```python
from build123d import *

# Parameters (mm, degrees)
SKETCH1_W                = 150
SKETCH1_H                = 12
BOSS_EXTRUDE1_DEPTH      = 20
SKETCH2_R                = 20
SKETCH2_R_2              = 10
BOSS_EXTRUDE2_DEPTH      = 30
FILLET1_R                = 10
SKETCH3_W                = 10
SKETCH3_H                = 80
BOSS_EXTRUDE3_DEPTH      = 15
BOSS_EXTRUDE4_DEPTH      = 40
BOSS_EXTRUDE4_DEPTH_BACK = 20
SKETCH4_R                = 15
SKETCH4_R_2              = 7.5
RIB1_START               = -5
RIB1_DEPTH               = 10


# Read off the part's stored shape, not the designer's step: Rib1
with BuildPart() as part:
    # Sketch1 → Boss-Extrude1 (new, symmetric)
    with BuildSketch(Plane.YZ):
        with Locations((75, 6)):
            Rectangle(SKETCH1_W, SKETCH1_H)
    extrude(amount=BOSS_EXTRUDE1_DEPTH, both=True)

    # Sketch2 → Boss-Extrude2 (add, symmetric)
    with BuildSketch(Plane.YZ):
        with Locations(Location((100, 30, 0), (0, 0, 270))):
            Circle(SKETCH2_R)
        with Locations(Location((100, 30, 0), (0, 0, 270))):
            Circle(SKETCH2_R_2, mode=Mode.SUBTRACT)
    extrude(amount=BOSS_EXTRUDE2_DEPTH, both=True)

    # Fillet1
    fillet1_edges = [part.edges().sort_by_distance(p)[0] for p in [
        (0, 108.717797887, 12),
    ]]
    fillet(fillet1_edges, radius=FILLET1_R)

    # Sketch3 → Boss-Extrude3 (add, symmetric)
    with BuildSketch(Plane.YZ):
        with Locations((35, 52)):
            Rectangle(SKETCH3_W, SKETCH3_H)
    extrude(amount=BOSS_EXTRUDE3_DEPTH, both=True)

    # Sketch4 → Boss-Extrude4 (add, two sides: drawn at the far end of the back side and taken through both)
    with BuildSketch(Plane(origin=(0, 40, 0), x_dir=(-1, 0, 0), z_dir=(0, 1, 0)).offset(-BOSS_EXTRUDE4_DEPTH_BACK)):
        with Locations(Location((0, 92, 0), (0, 0, 90))):
            Circle(SKETCH4_R)
        with Locations(Location((0, 92, 0), (0, 0, 90))):
            Circle(SKETCH4_R_2, mode=Mode.SUBTRACT)
    extrude(amount=BOSS_EXTRUDE4_DEPTH + BOSS_EXTRUDE4_DEPTH_BACK)

    # Rib1 outline → Rib1 (add)
    with BuildSketch(Plane.YZ.offset(RIB1_START)):
        with BuildLine():
            ThreePointArc((85, 50), (81.464466094, 51.464466094), (80, 55))
            Line((80, 55), (80, 79))
            Line((80, 79), (40, 79))
            Line((40, 79), (40, 12))
            Line((40, 12), (91.282202113, 12))
            ThreePointArc((91.282202113, 12), (80.50641131, 34.472135955), (100, 50))
            Line((100, 50), (85, 50))
        make_face()
    extrude(amount=RIB1_DEPTH)


solid = part.part
```
Geometry: final body of the model. Coordinates: model frame, mm. A direction names the side the tool comes from. Give positions to 0.01 mm unless a question says otherwise; leave off trailing zeros. Order: outer loops, then holes, each group sorted by start corner. A loop starts at its lowest first (then second) coordinate and runs counter-clockwise, first axis right, second up. Notation, with made-up numbers: (74, -34.5) -> (88, -34.5) arc R26 cw to (88, -18.5) -> close; hole circle Ø4 at (89.5, 62). An arc over 180 degrees is marked (long way). Write each question's results on one line, items separated by ' | '. Start each with the question number.
1) Section B-B (x = 0). Return loops of the section in (y, z).
2) Section D-D (z = 67). Return loops of the section in (x, y), then the cut area to 3 significant figures.
3) Line query: line 1 (Y direction, x = -8, z = 30); line 2 (Z direction, x = 0, y = 67); line 3 (X direction, y = 62.5, z = 92). Output: solid intervals per line, ascending. Write a range as from..to.
4) Section C-C (y = 76). Return loops of the section in (x, z), then the cut area to 3 significant figures.
5) Section A-A (y = 24). Return loops of the section in (x, z), then the cut area to 3 significant figures.
6) Set-up query: faces 4 (the cylindrical face through (-5.745, 49.58, 105.856)), 5 (the flat face through (10, 40, 51)), 6 (the flat face through (-15, 35, 53)), 7 (the flat face through (0, 35, 92)), 8 (the flat face through (0, 93, 50)). Return all of +Z, -Z, +X, -X, +Y, -Y with unobstructed straight access to the full face (end or side cutting, diameter ignored); none if empty.
7) Draft query along Y for faces 1 (the flat face through (15, 35, 53)), 2 (the cylindrical face through (0.42, 100.88, 49.98)), 3 (the flat face through (0, 150, 6)). Return one class per face: pulls with the +Y half, pulls with the -Y half, needs draft (parallel to the pull), parting line crosses it, or undercut.
8) First-contact query: pin 1 (1.5 mm diameter, centred on x = 12.5, y = 31.5, fed in from -Z); pin 2 (8 mm diameter, centred on y = 34.5, z = 63.5, fed in from -X); pin 3 (1.5 mm diameter, centred on x = 6, z = 45, fed in from -Y); pin 4 (8 mm diameter, centred on x = -1, y = 95.5, fed in from +Z). Flat tips, straight axial feed; report the tip coordinate or a pass-through.
Calculated:
1) outline: (0, 0) -> (150, 0) -> (150, 12) -> (128.91, 12) arc R10 cw to (119.28, 24.67) arc R20 ccw to (100, 50) -> (85, 50) arc R5 cw to (80, 55) -> (80, 84.5) -> (40, 84.5) -> (40, 92) -> (30, 92) -> (30, 84.5) -> (20, 84.5) -> (20, 77) -> (30, 77) -> (30, 12) -> (0, 12) -> close; (20, 99.5) -> (80, 99.5) -> (80, 107) -> (20, 107) -> close; hole circle Ø20 at (100, 30)
2) outline: (-15, 30) -> (15, 30) -> (15, 40) -> (5, 40) -> (5, 80) -> (-5, 80) -> (-5, 40) -> (-15, 40) -> close | area: 700 mm2
3) line 1: 30..40, 80..90, 110..120 | line 2: 0..84.5, 99.5..107 | line 3: -15..-7.5, 7.5..15
4) outline: (-20, 0) -> (20, 0) -> (20, 12) -> (5, 12) -> (5, 77.86) arc R15 ccw (long way) to (-5, 77.86) -> (-5, 12) -> (-20, 12) -> close; hole circle Ø15 at (0, 92) | area: 1,660 mm2
5) outline: (-20, 0) -> (20, 0) -> (20, 12) -> (-20, 12) -> close; circle Ø30 at (0, 92); hole circle Ø15 at (0, 92) | area: 1,010 mm2
6) face 4: none | face 5: +X | face 6: +Z, -X, -Y | face 7: +Y, -Y | face 8: +Z, +X, -X, +Y
7) face 1: needs draft | face 2: undercut | face 3: pulls with the +Y half
8) pin 1: z = 0 | pin 2: x = -15 | pin 3: y = 30 | pin 4: z = 50
